from build123d import *

# Parameters (mm, degrees)
F0_R     = 11.1
F1_DEPTH = 7


with BuildPart() as f1:
    # F0 (on Top) → F1 (new body)
    with BuildSketch(Plane.XY):
        with BuildLine():
            ThreePointArc((13.696931, 25.102746), (11.974288, 27.214871), (13.957972, 29.083981))
            ThreePointArc((13.957972, 29.083981), (13.9413, 29.280684), (13.921856, 29.477133))
            ThreePointArc((13.921856, 29.477133), (11.630843, 30.953557), (12.939852, 33.344177))
            ThreePointArc((12.939852, 33.344177), (12.863211, 33.526101), (12.784013, 33.706927))
            ThreePointArc((12.784013, 33.706927), (10.148889, 34.403128), (10.655089, 37.081249))
            ThreePointArc((10.655089, 37.081249), (10.525982, 37.230586), (10.394781, 37.378087))
            ThreePointArc((10.394781, 37.378087), (7.673492, 37.225916), (7.327332, 39.929384))
            ThreePointArc((7.327332, 39.929384), (7.158396, 40.031516), (6.988036, 40.131255))
            ThreePointArc((6.988036, 40.131255), (4.44696, 39.145607), (3.282324, 41.609789))
            ThreePointArc((3.282324, 41.609789), (3.090096, 41.654717), (2.897254, 41.696931))
            ThreePointArc((2.897254, 41.696931), (0.785129, 39.974288), (-1.083981, 41.957972))
            ThreePointArc((-1.083981, 41.957972), (-1.280684, 41.9413), (-1.477133, 41.921856))
            ThreePointArc((-1.477133, 41.921856), (-2.953557, 39.630843), (-5.344177, 40.939852))
            ThreePointArc((-5.344177, 40.939852), (-5.526101, 40.863211), (-5.706927, 40.784013))
            ThreePointArc((-5.706927, 40.784013), (-6.403128, 38.148889), (-9.081249, 38.655089))
            ThreePointArc((-9.081249, 38.655089), (-9.230586, 38.525982), (-9.378087, 38.394781))
            ThreePointArc((-9.378087, 38.394781), (-9.225916, 35.673492), (-11.929384, 35.327332))
            ThreePointArc((-11.929384, 35.327332), (-12.031516, 35.158396), (-12.131255, 34.988036))
            ThreePointArc((-12.131255, 34.988036), (-11.145607, 32.44696), (-13.609789, 31.282324))
            ThreePointArc((-13.609789, 31.282324), (-13.654717, 31.090096), (-13.696931, 30.897254))
            ThreePointArc((-13.696931, 30.897254), (-11.974288, 28.785129), (-13.957972, 26.916019))
            ThreePointArc((-13.957972, 26.916019), (-13.852658, 25.974198), (-13.683867, 25.041659))
            ThreePointArc((-13.683867, 25.041659), (-16.468709, 7.258906), (-30.476603, -4.044214))
            ThreePointArc((-30.476603, -4.044214), (-30.506332, -4.053796), (-30.536039, -4.063444))
            ThreePointArc((-30.536039, -4.063444), (-31.503871, -6.611359), (-34.114409, -5.827993))
            ThreePointArc((-34.114409, -5.827993), (-34.276424, -5.940783), (-34.436831, -6.055846))
            ThreePointArc((-34.436831, -6.055846), (-34.569945, -8.778134), (-37.294788, -8.839809))
            Line((-37.294788, -8.839809), (-37.531019, -9.156145))
            ThreePointArc((-37.531019, -9.156145), (-36.816385, -11.786329), (-39.388805, -12.687008))
            ThreePointArc((-39.388805, -12.687008), (-39.453581, -12.873487), (-39.515721, -13.06086))
            ThreePointArc((-39.515721, -13.06086), (-38.023292, -15.34148), (-40.191484, -16.992998))
            ThreePointArc((-40.191484, -16.992998), (-40.195465, -17.190367), (-40.196662, -17.387772))
            ThreePointArc((-40.196662, -17.387772), (-38.072527, -19.095584), (-39.624253, -21.33628))
            ThreePointArc((-39.624253, -21.33628), (-39.567049, -21.525218), (-39.507186, -21.713332))
            ThreePointArc((-39.507186, -21.713332), (-36.959271, -22.681164), (-37.742637, -25.291702))
            ThreePointArc((-37.742637, -25.291702), (-37.629847, -25.453716), (-37.514784, -25.614124))
            ThreePointArc((-37.514784, -25.614124), (-34.792496, -25.747238), (-34.730821, -28.472081))
            ThreePointArc((-34.730821, -28.472081), (-34.573486, -28.591311), (-34.414485, -28.708311))
            ThreePointArc((-34.414485, -28.708311), (-31.784301, -27.993677), (-30.883622, -30.566098))
            ThreePointArc((-30.883622, -30.566098), (-30.697143, -30.630874), (-30.50977, -30.693014))
            ThreePointArc((-30.50977, -30.693014), (-28.22915, -29.200585), (-26.577632, -31.368777))
            Line((-26.577632, -31.368777), (-26.182858, -31.373954))
            ThreePointArc((-26.182858, -31.373954), (-24.475046, -29.24982), (-22.23435, -30.801546))
            ThreePointArc((-22.23435, -30.801546), (-22.045412, -30.744341), (-21.857298, -30.684478))
            ThreePointArc((-21.857298, -30.684478), (-20.889466, -28.136563), (-18.278928, -28.919929))
            ThreePointArc((-18.278928, -28.919929), (-17.515944, -28.357813), (-16.792736, -27.745367))
            ThreePointArc((-16.792736, -27.745367), (0, -21.265734), (16.792736, -27.745367))
            ThreePointArc((16.792736, -27.745367), (16.815899, -27.766322), (16.839108, -27.787225))
            ThreePointArc((16.839108, -27.787225), (19.529583, -27.351435), (20.156437, -30.00391))
            ThreePointArc((20.156437, -30.00391), (20.335123, -30.087823), (20.514975, -30.169209))
            ThreePointArc((20.514975, -30.169209), (22.939103, -28.923345), (24.354936, -31.25229))
            Line((24.354936, -31.25229), (24.747006, -31.298705))
            ThreePointArc((24.747006, -31.298705), (26.667495, -29.364721), (28.733716, -31.142163))
            ThreePointArc((28.733716, -31.142163), (28.9276, -31.105022), (29.12094, -31.06515))
            ThreePointArc((29.12094, -31.06515), (30.3498, -28.632358), (32.864153, -29.684309))
            ThreePointArc((32.864153, -29.684309), (33.037069, -29.589072), (33.208626, -29.491406))
            ThreePointArc((33.208626, -29.491406), (33.625567, -26.797945), (36.34193, -27.021431))
            ThreePointArc((36.34193, -27.021431), (36.476953, -26.877421), (36.609932, -26.731522))
            ThreePointArc((36.609932, -26.731522), (36.174142, -24.041046), (38.826617, -23.414193))
            Line((38.826617, -23.414193), (38.991916, -23.055655))
            ThreePointArc((38.991916, -23.055655), (37.691962, -20.885304), (39.558538, -19.177617))
            Line((39.558538, -19.177617), (39.558538, -18.723724))
            ThreePointArc((39.558538, -18.723724), (38.196729, -16.616714), (39.964871, -14.836913))
            ThreePointArc((39.964871, -14.836913), (39.927729, -14.64303), (39.887857, -14.44969))
            ThreePointArc((39.887857, -14.44969), (37.455066, -13.22083), (38.507016, -10.706477))
            ThreePointArc((38.507016, -10.706477), (38.411779, -10.533561), (38.314113, -10.362004))
            ThreePointArc((38.314113, -10.362004), (35.620652, -9.945063), (35.844139, -7.2287))
            ThreePointArc((35.844139, -7.2287), (35.700129, -7.093677), (35.554229, -6.960698))
            ThreePointArc((35.554229, -6.960698), (32.863754, -7.396488), (32.2369, -4.744012))
            ThreePointArc((32.2369, -4.744012), (31.368601, -4.364307), (30.476603, -4.044214))
            ThreePointArc((30.476603, -4.044214), (16.55242, 7.115022), (13.615685, 24.71579))
            ThreePointArc((13.615685, 24.71579), (13.612737, 24.716735), (13.609789, 24.717676))
            ThreePointArc((13.609789, 24.717676), (13.647789, 24.879448), (13.683867, 25.041659))
            ThreePointArc((13.683867, 25.041659), (13.690433, 25.072195), (13.696931, 25.102746))
        make_face()
        with Locations((-26.196669, -17.373961)):
            Circle(F0_R, mode=Mode.SUBTRACT)
        with Locations((26.196669, -17.373961)):
            Circle(F0_R, mode=Mode.SUBTRACT)
        Circle(F0_R, mode=Mode.SUBTRACT)
        with Locations((0, 28)):
            Circle(F0_R, mode=Mode.SUBTRACT)
        with BuildLine():
            ThreePointArc((13.615685, 24.71579), (13.649233, 24.878838), (13.683867, 25.041659))
            ThreePointArc((13.683867, 25.041659), (13.647789, 24.879448), (13.609789, 24.717676))
            ThreePointArc((13.609789, 24.717676), (13.612737, 24.716735), (13.615685, 24.71579))
        make_face()
        with BuildLine():
            ThreePointArc((40.121412, -18.823624), (39.836387, -18.793889), (39.558538, -18.723724))
            Line((39.558538, -18.723724), (39.558538, -19.177617))
            ThreePointArc((39.558538, -19.177617), (39.818006, -19.179869), (40.074998, -19.215694))
            ThreePointArc((40.074998, -19.215694), (40.099587, -19.019823), (40.121412, -18.823624))
        make_face()
    extrude(amount=F1_DEPTH)


solid = f1.part
The model under review builds one solid part; all positions refer to its coordinate system, in mm. Round coordinates to 2 decimals unless told otherwise and drop trailing zeros. Loops run counter-clockwise (first coordinate to the right, second up) from the corner with the lowest first, then second, coordinate; pieces in that order, holes last. Notation, with made-up numbers: M 61,64 L 66,64 A23 ccw 66,101 Z; hole C -33.75,73 d11. An arc over 180 degrees is marked long. Answer as CSV lines item,"result".
1. We need section A-A (x = 0.5). Give the boundary of the cut face in (y, z), plus the area to 3 significant figures.
Outcome:
outline,"M -21.27,0 L -11.09,0 L -11.09,7 L -21.27,7 Z; M 11.09,0 L 16.91,0 L 16.91,7 L 11.09,7 Z; M 39.09,0 L 40.01,0 L 40.01,7 L 39.09,7 Z"
area,"119 mm2"
2. We need section D-D (z = 3.5). Count the separate pieces of the cut face and the enclosed holes in it, plus the area to 3 significant figures.
Outcome:
separate pieces,"1"
enclosed holes,"4"
area,"1,380 mm2"
3. To check wall thickness, follow L1, parallel to X at y = -20, z = 5.75; L2, parallel to X at y = 38, z = 4.25; L3, parallel to X at y = -9.5, z = 3. State the ranges of each line that lie inside material, in increasing order. Write a range as [from, to].
Outcome:
L1,"x = [-38.15, -36.98], [-15.41, 15.41], [36.98, 38.05]"
L2,"x = [-9.06, -8.25], [-6.69, -4.82], [4.82, 7.1]"
L3,"x = [-37.12, -34.02], [-18.37, -5.74], [5.74, 18.37], [34.02, 35.36]"
4. We need section B-B (y = 28). Give the boundary of the cut face in (x, z), plus the area to 3 significant figures.
Outcome:
outline,"M -12.19,0 L -11.1,0 L -11.1,7 L -12.19,7 Z; M 11.1,0 L 12.19,0 L 12.19,7 L 11.1,7 Z"
area,"15.3 mm2"
5. We need section C-C (x = -20). Give the boundary of the cut face in (y, z).
Outcome:
outline,"M -27.93,0 L -26.58,0 L -26.58,7 L -27.93,7 Z; M -8.16,0 L 2.53,0 L 2.53,7 L -8.16,7 Z"
6. Draft analysis for pull direction Y (two halves, no side actions). For faces 1 (the face through (10.17, 34.37, 3.45)), 2 (the face through (4.49, 39.13, 3.45)), 3 (the face through (0.83, 39.97, 3.45)), 4 (the face through (-0.258, -21.267, 3.451)), state which applies: pulls with the +Y half, pulls with the -Y half, needs draft (parallel to the pull), parting line crosses it, or undercut.
Outcome:
face 1,"undercut"
face 2,"undercut"
face 3,"pulls with the +Y half"
face 4,"pulls with the -Y half"
7. Insertion check: pin 1 Ø20 at (x, y) = (-26.2, -17.37) entering from +Z. The pin has a flat end and moves straight along its axis. Give the tip position at first contact, or say it passes through.
Outcome:
pin 1,"passes through"
